Design review of the part built by this model. Coordinates are the model's own, in mm. A direction names the side the tool comes from. Coordinates: 2 decimals unless noted, no trailing zeros. Write each loop counter-clockwise with the first axis right and the second up, starting at its lowest first coordinate (ties: lowest second). Pieces come first, ordered by that corner, then holes.
Q1. Take a section at C-C (z = 18). Give the boundary of the cut face in (x, y), and give its area (3 significant figures).
Q2. For probe 1 along X at (y, z) = (-2, 0) (3 decimals); probe 2 along Z at (x, y) = (15, 24); probe 3 along X at (y, z) = (2.5, -1), list the stretches that pass through material, from the lowest coordinate up.
Q3. Take a section at B-B (x = 18). Give the boundary of the cut face in (y, z), and give its area (3 significant figures).
Q4. Insertion check: pin 1 (3.5 mm diameter, centred on x = 1, z = -13, fed in from +Y); pin 2 (3 mm diameter, centred on x = 4, y = 25.5, fed in from +Z); pin 3 (13 mm diameter, centred on x = -1.53, z = -13.89, fed in from +Y); pin 4 (5 mm diameter, centred on x = 14.5, z = 16, fed in from -Y). Each pin has a flat end and moves straight along its axis. Give the tip position at first contact, or say it passes through.
Q5. Mouldability with a two-part tool opening along X and no side actions: class faces 4 (the cylindrical face through (2.861, 4.383, 9.085)), 5 (the flat face through (-14, 23.178, 1)), 6 (the flat face through (7, 8.89, 7)) as pulls with the +X half, pulls with the -X half, needs draft (parallel to the pull), parting line crosses it, or undercut.
Q6. Take a section at D-D (z = -13). Give the boundary of the cut face in (x, y), and give its area (3 significant figures).
Q7. Machinability: for faces 1 (the flat face through (0, 10.16, 0)), 2 (the flat face through (2.2, -5.08, 2.2)), 3 (the cylindrical face through (-1.286, 28.812, -19.437)), which of the approach directions +Z, -Z, +X, -X, +Y, -Y give a long, thin tool a straight path to every point of the face, cutting with its end or side? Answer none if there is none.
```python
from build123d import *

# Parameters (mm, degrees)
SKETCH_1_R          = 9.525
EXTRUDE_1_DEPTH     = 16.51
SKETCH_2_R          = 22.86
EXTRUDE_2_DEPTH     = 17.78
CUT_EXTRUDE_1_DEPTH = 10.16
SKETCH_3_R          = 5.55625
CUT_EXTRUDE_2_DEPTH = 11.1125
SKETCH_5_R          = 1.55
CUT_EXTRUDE_3_DEPTH = 32
SKETCH_6_W          = 7.62
SKETCH_6_H          = 7.62
EXTRUDE_START       = 5.08
SKETCH_7_R          = 5.08
EXTRUDE_3_DEPTH     = 5.08


with BuildPart() as part:
    # 草图1 → 凸台-拉伸1 (new body)
    with BuildSketch(Plane(origin=(0, 0, 0), x_dir=(1, 0, 0), z_dir=(0, 1, 0))):
        with Locations(Location((0, 0, 0), (0, 0, 270))):
            Circle(SKETCH_1_R)
    extrude(amount=EXTRUDE_1_DEPTH)

    # 草图2 → 凸台-拉伸2 (add)
    with BuildSketch(Plane(origin=(0, 16.51, 0), x_dir=(1, 0, 0), z_dir=(0, 1, 0))):
        with Locations(Location((0, 0, 0), (0, 0, 270))):
            Circle(SKETCH_2_R)
    extrude(amount=EXTRUDE_2_DEPTH)

    # 草图4 → 切除-拉伸1 (cut)
    with BuildSketch(Plane.XZ):
        with BuildLine():
            Line((3.080497473, 0.768869508), (0.87438821, 3.052223822))
            ThreePointArc((0.87438821, 3.052223822), (-2.283354313, -2.206109263), (3.080497473, 0.768869508))
        make_face()
    extrude(amount=-CUT_EXTRUDE_1_DEPTH, mode=Mode.SUBTRACT)

    # 草图3 → 切除-拉伸2 (cut)
    with BuildSketch(Plane(origin=(0, 34.29, 0), x_dir=(1, 0, 0), z_dir=(0, 1, 0))):
        with Locations(Location((-13.885899292, -1.530588399, 0), (0, 0, 270))):
            Circle(SKETCH_3_R)
        with Locations(Location((-1.530588399, 13.885899292, 0), (0, 0, 270))):
            Circle(SKETCH_3_R)
        with Locations(Location((13.885899292, 1.530588399, 0), (0, 0, 270))):
            Circle(SKETCH_3_R)
        with Locations(Location((1.530588399, -13.885899292, 0), (0, 0, 270))):
            Circle(SKETCH_3_R)
    extrude(amount=-CUT_EXTRUDE_2_DEPTH, mode=Mode.SUBTRACT)

    # 草图5 → 切除-拉伸3 (cut)
    with BuildSketch(Plane(origin=(-7.155974413, 0, -6.913890386), x_dir=(-0.6948375630636291, 0, 0.7191667129086254), z_dir=(-0.7191667129086254, 0, -0.6948375630636291))):
        with Locations((0, 5.08)):
            Circle(SKETCH_5_R)
    extrude(amount=-CUT_EXTRUDE_3_DEPTH, mode=Mode.SUBTRACT)

    # 草图6 → 旋转2 (revolve)
    with BuildSketch(Plane(origin=(0, 0, 0), x_dir=(-0.9998520121667556, 0, 0.01720330683589877), z_dir=(-0.01720330683589877, 0, -0.9998520121667556)), mode=Mode.PRIVATE) as revolve_2_sk:
        with Locations((-13.335, 12.7)):
            Rectangle(SKETCH_6_W, SKETCH_6_H)
    revolve(revolve_2_sk.sketch.rotate(Axis((0, 16.51, 0), (0, -1, 0)), 90.985725501), axis=Axis((0, 16.51, 0), (0, -1, 0)))

    # 草图7 → 凸台-拉伸3 (add)
    with BuildSketch(Plane.XZ.offset(EXTRUDE_START)):
        with Locations(Location((0, 0, 0), (0, 0, 90))):
            Circle(SKETCH_7_R)
        with BuildLine():
            Line((0.87438821, 3.052223822), (3.080497473, 0.768869508))
            ThreePointArc((3.080497473, 0.768869508), (-2.283354313, -2.206109263), (0.87438821, 3.052223822))
        make_face(mode=Mode.SUBTRACT)
    extrude(amount=-EXTRUDE_3_DEPTH)


solid = part.part
```
Response:
1. outline: (-14.09, 16.51) - (14.09, 16.51) - (14.09, 34.29) - (5.27, 34.29) - (5.27, 23.18) - (-2.2, 23.18) - (-2.2, 34.29) - (-14.09, 34.29) - close
1. area: 418 mm2
2. probe 1: x = -5.08 to -3.175, 3.175 to 5.08
2. probe 2: z = -17.25 to -6.97, 3.91 to 17.25
2. probe 3: x = -9.47 to -3.01, 3.01 to 9.47
3. outline: (16.51, -14.09) - (34.29, -14.09) - (34.29, -5.27) - (23.18, -5.27) - (23.18, 2.2) - (34.29, 2.2) - (34.29, 14.09) - (16.51, 14.09) - close
3. area: 418 mm2
4. pin 1: stops at y = 23.18
4. pin 2: stops at z = 22.72
4. pin 3: stops at y = 34.29
4. pin 4: stops at y = 16.51
5. face 4: parting line crosses it
5. face 5: undercut
5. face 6: needs draft
6. outline: (-18.8, 16.51) - (-11.18, 16.51) - (-11.18, 8.89) - (11.18, 8.89) - (11.18, 16.51) - (18.8, 16.51) - (18.8, 34.29) - (3.95, 34.29) - (3.95, 23.18) - (-7.02, 23.18) - (-7.02, 34.29) - (-18.8, 34.29) - close
6. area: 717 mm2
7. face 1: -Y
7. face 2: +Z, -Z, +X, -X, -Y
7. face 3: +Y
